The listing builds one solid part. Answer for the finished solid, in the listing's coordinates (mm). Face numbers are marked on the shaded views. Round coordinates to 2 decimals unless told otherwise and drop trailing zeros. Order: outer loops, then holes, each group sorted by start corner. A loop starts at its lowest first (then second) coordinate and runs counter-clockwise, first axis right, second up. Notation, with made-up numbers: M -27,54 L 12,54 A18 cw 12,77 Z; hole C 52.25,74.25 d5. An arc over 180 degrees is marked long. Write item = value, one per line. Start each with the question number.
(1) A cutting plane is placed at C-C, the plane z = 22.5. Determine the outline of the cut face in (x, y).
(2) Each of these flat-tipped pins is pushed along its axis until it touches: pin 1 (10 mm diameter, centred on y = 8.5, z = 14, fed in from -X); pin 2 (8 mm diameter, centred on x = -7, y = 26.5, fed in from +Z). Where does it stop, or does it pass through?
(3) Straight lines are drawn through the part: probe 1 along Y at (x, z) = (0, 2.35); probe 2 along Y at (x, z) = (33, 1.5); probe 3 along Y at (x, z) = (-25.5, 2.25). For each, find the intervals that lie inside material, in ascending order. Write a range as from..to.
(4) A cutting plane is placed at A-A, the plane x = 0. Determine the outline of the cut face in (y, z).
(5) A cutting plane is placed at D-D, the plane x = -33. Determine the outline of the cut face in (y, z), and give its area (3 significant figures).
(6) For a pull along Y with two mould halves and no side action, classify the marked faces 1, 2 and 3 as released by +Y, released by -Y, zero draft, split by the parting line, or undercut.
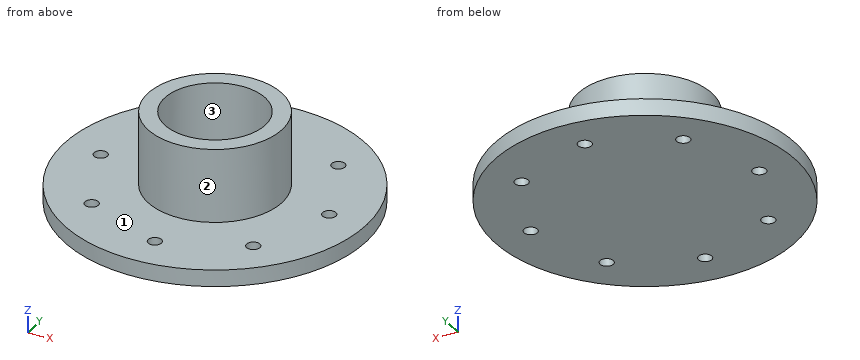
from build123d import *

# Parameters (mm, degrees)
SKETCH_1_R          = 45
EXTRUDE_1_DEPTH     = 5
SKETCH_2_R          = 20
SKETCH_2_R_2        = 15
EXTRUDE_2_DEPTH     = 22
SKETCH_3_R          = 2
CUT_EXTRUDE_3_DEPTH = 68.334983478


with BuildPart() as part:
    # Эскиз1 → Вытянуть1 (new body)
    with BuildSketch(Plane.XY):
        Circle(SKETCH_1_R)
    extrude(amount=EXTRUDE_1_DEPTH)

    # Эскиз2 → Вытянуть2 (add)
    with BuildSketch(Plane.XY.offset(5)):
        Circle(SKETCH_2_R)
        Circle(SKETCH_2_R_2, mode=Mode.SUBTRACT)
    extrude(amount=EXTRUDE_2_DEPTH)

    # Эскиз3 → Вытянуть3 (cut, through all)
    with BuildSketch(Plane.XY.offset(5)):
        with Locations((0, 33.781150957)):
            Circle(SKETCH_3_R)
        with Locations((23.886880918, 23.886880918)):
            Circle(SKETCH_3_R)
        with Locations((33.781150957, 0)):
            Circle(SKETCH_3_R)
        with Locations((23.886880918, -23.886880918)):
            Circle(SKETCH_3_R)
        with Locations((0, -33.781150957)):
            Circle(SKETCH_3_R)
        with Locations((-23.886880918, -23.886880918)):
            Circle(SKETCH_3_R)
        with Locations((-33.781150957, 0)):
            Circle(SKETCH_3_R)
        with Locations((-23.886880918, 23.886880918)):
            Circle(SKETCH_3_R)
    extrude(amount=-CUT_EXTRUDE_3_DEPTH, mode=Mode.SUBTRACT)


solid = part.part
Reported:
q1.outline = C 0,0 d40; hole C 0,0 d30
q2.pin_1 = -19.69
q2.pin_2 = 5
q3.probe_1 = -45..-35.78, -31.78..31.78, 35.78..45
q3.probe_2 = -30.59..-1.84, 1.84..30.59
q3.probe_3 = -37.08..-25.07, -22.7..22.7, 25.07..37.08
q4.outline = M -45,0 L -35.78,0 L -35.78,5 L -45,5 Z; M -31.78,0 L 31.78,0 L 31.78,5 L 20,5 L 20,27 L 15,27 L 15,5 L -15,5 L -15,27 L -20,27 L -20,5 L -31.78,5 Z; M 35.78,0 L 45,0 L 45,5 L 35.78,5 Z
q5.outline = M -30.59,0 L -1.84,0 L -1.84,5 L -30.59,5 Z; M 1.84,0 L 30.59,0 L 30.59,5 L 1.84,5 Z
q5.area = 288 mm²
q6.face_1 = zero draft
q6.face_2 = split by the parting line
q6.face_3 = undercut
